Could you check a few things on this model? Use its own coordinates, in mm. A direction names the side the tool comes from. Give positions to 0.01 mm unless a question says otherwise; leave off trailing zeros. Loops run counter-clockwise (first coordinate to the right, second up) from the corner with the lowest first, then second, coordinate; pieces in that order, holes last. Notation, with made-up numbers: M -36.5,63 L 15.5,63 A18 ccw 15.5,82 Z; hole C 38.25,22.5 d1. An arc over 180 degrees is marked long. Answer in a Markdown table with one row per item. Add a question column.
1. If we section it at C-C on z = -2.5: List the corners of the cut face in (x, y) for me, then the cut area to 3 significant figures.
2. Thinking about a two-plate mould opening in X: for faces 1 (the flat face through (-9.798, 4.583, 0.305)), 2 (the cylindrical face through (-6.96, 6.08, 4.26)), 3 (the conical face through (12.598, 7.766, 4.651)), 4 (the cylindrical face through (-0.728, 1.479, 1.755)), which applies, released by +X, released by -X, zero draft, split by the parting line, or undercut?
3. Which directions (+Z, -Z, +X, -X, +Y, -Y) give clear straight access to the entire face, cutting with the end or side of a thin tool? Please do faces 5 (the flat face through (0, 8, -6)), 6 (the cylindrical face through (-4.064, 1.682, -17.022)), 7 (the flat face through (17, 2, 1.333)), 8 (the flat face through (-7.11, 2.06, -14.98)).
4. If we section it at D-D on y = 6.5: List the corners of the cut face in (x, z) for me.
5. If we section it at A-A on x = 0: List the corners of the cut face in (y, z) for me.
6. I need wall thicknesses on line 1 along Y through (x, z) = (2, 5); line 2 along Z through (x, y) = (1.5, 6.25); line 3 along Z through (x, y) = (-2, 4.75). Which ranges of each line are inside material? Lowest first, please. Write a range as from..to.
7. If we section it at B-B on y = 9: List the corners of the cut face in (x, z) for me.
8. I'm going to push flat-ended pins straight in: pin 1 Ø3.5 at (x, y) = (-1.5, 8.5) entering from -Z; pin 2 Ø3 at (y, z) = (7, 3) entering from +X; pin 3 Ø3 at (x, y) = (4.5, 6) entering from -Z; pin 4 Ø2.5 at (x, z) = (0, 0) entering from +Y. Where does each tip first touch, or does it pass through?
```python
from build123d import *

# Parameters (mm, degrees)
SKETCH1_R           = 1.9
BOSS_EXTRUDE1_DEPTH = 12
CIRPATTERN1_COUNT   = 3
CUT_EXTRUDE1_DEPTH  = 9
SKETCH4_R           = 1.9
CUT_EXTRUDE2_DEPTH  = 12
CIRPATTERN2_COUNT   = 3


with BuildPart() as part:
    # Sketch1 → Boss-Extrude1 (new body)
    with BuildSketch(Plane(origin=(0, 0, 0), x_dir=(1, 0, 0), z_dir=(0, 1, 0))):
        with BuildLine():
            ThreePointArc((-0.477365515, 17.493487993), (-4.114019559, 17.009551525), (-7.569865672, 15.778058617))
            Line((-7.569865672, 15.778058617), (-6.639528096, 14.166666667))
            ThreePointArc((-6.639528096, 14.166666667), (-5.43375673, 9.666666667), (-6.639528096, 5.166666667))
            Line((-6.639528096, 5.166666667), (-14.43375673, -8.333333333))
            Line((-14.43375673, -8.333333333), (14.43375673, -8.333333333))
            Line((14.43375673, -8.333333333), (-0.477365515, 17.493487993))
        make_face()
        with Locations(Location((0, 0, 0), (0, 0, 270))):
            Circle(SKETCH1_R, mode=Mode.SUBTRACT)
    boss_extrude1 = extrude(amount=BOSS_EXTRUDE1_DEPTH)

    # CirPattern1: Boss-Extrude1 ×3 about axis
    cirpattern1_axis = Axis((0, 0, 0), (0, 1, 0))
    for i in range(1, CIRPATTERN1_COUNT):
        add(boss_extrude1.rotate(cirpattern1_axis, i * 360 / CIRPATTERN1_COUNT))

    # Sketch3 → Cut-Extrude1 (cut)
    with BuildSketch(Plane(origin=(0, 12, 0), x_dir=(1, 0, 0), z_dir=(0, 1, 0))):
        Polygon((3.464101615, 6), (-3.464101615, 6), (-6.92820323, 0), (-3.464101615, -6), (3.464101615, -6), (6.92820323, 0), align=None)
    extrude(amount=-CUT_EXTRUDE1_DEPTH, mode=Mode.SUBTRACT)

    # Sketch4 → Cut-Extrude2 (cut)
    with BuildSketch(Plane(origin=(0, 12, 0), x_dir=(1, 0, 0), z_dir=(0, 1, 0))):
        with Locations(Location((-0.780031957, 9.96953109, 0), (0, 0, 270))):
            Circle(SKETCH4_R)
    cut_extrude2 = extrude(amount=-CUT_EXTRUDE2_DEPTH, mode=Mode.SUBTRACT)

    # CirPattern2: Cut-Extrude2 ×3 about axis
    cirpattern2_axis = Axis((0, 0, 0), (0, 1, 0))
    for i in range(1, CIRPATTERN2_COUNT):
        add(cut_extrude2.rotate(cirpattern2_axis, i * 360 / CIRPATTERN2_COUNT), mode=Mode.SUBTRACT)

    # Sketch5 → Cut-Revolve2 (revolve, cut)
    with BuildSketch(Plane.XY):
        Polygon((17.884587384, 3), (9.470286093, 12), (17.884587384, 12), align=None)
    revolve(axis=Axis((0, 0, 0), (0, 1, 0)), mode=Mode.SUBTRACT)


solid = part.part
```
Results:
| question | item | result |
|---|---|---|
| 1 | outline | M -8.18,0 L 8.22,0 L 8.22,12 L 5.48,12 L 5.48,3 L -5.48,3 L -5.48,12 L -8.18,12 Z |
| 1 | area | 98.1 mm2 |
| 2 | face 1 | released by -X |
| 2 | face 2 | undercut |
| 2 | face 3 | released by +X |
| 2 | face 4 | undercut |
| 3 | face 5 | +Y |
| 3 | face 6 | -Z, -X, +Y, -Y |
| 3 | face 7 | -Z, +X, +Y, -Y |
| 3 | face 8 | -X, +Y, -Y |
| 4 | outline | M -13.22,6.23 L -6.64,-5.17 A9 cw -6.18,-13.24 A14.61 ccw 1.22,-14.56 L 7.79,-3.17 A9 cw 14.56,1.27 A14.61 ccw 12,8.33 L -1.15,8.33 A9 cw -8.38,11.97 A14.61 ccw Z; hole C -8.24,5.66 d3.8; hole M -6.93,0 L -3.46,-6 L 3.46,-6 L 6.93,0 L 3.46,6 L -3.46,6 Z; hole C -0.78,-9.97 d3.8; hole C 9.02,4.31 d3.8 |
| 5 | outline | M 0,-16.67 L 4.3,-16.67 L 9.61,-11.7 L 0,-11.7 Z; M 0,-8.24 L 12,-8.24 L 12,-6 L 3,-6 L 3,-1.9 L 0,-1.9 Z; M 0,1.9 L 3,1.9 L 3,6 L 12,6 L 12,8.33 L 0,8.33 Z |
| 6 | line 1 | 0..3 |
| 6 | line 2 | -14.07..-6, 6..8.33 |
| 6 | line 3 | -16.12..-11.43, -8.51..-6, 6..8.37 |
| 7 | outline | M -11.72,3.64 L -6.64,-5.17 A9 cw -5.53,-10.96 A12.28 ccw 2.71,-11.97 L 7.79,-3.17 A9 cw 12.26,0.69 A12.28 ccw 9.01,8.33 L -1.15,8.33 A9 cw -6.73,10.27 A12.28 ccw Z; hole C -8.24,5.66 d3.8; hole M -6.93,0 L -3.46,-6 L 3.46,-6 L 6.93,0 L 3.46,6 L -3.46,6 Z; hole C -0.78,-9.97 d3.8; hole C 9.02,4.31 d3.8 |
| 8 | pin 1 | z = -14.31 |
| 8 | pin 2 | x = 15.28 |
| 8 | pin 3 | z = -11.47 |
| 8 | pin 4 | through |
